Source: CAD feature listing. Evaluate the final solid. Frame: model axes, mm. A direction names the side the tool comes from. Give positions to 0.01 mm unless a question says otherwise; leave off trailing zeros. Loops run counter-clockwise (first coordinate to the right, second up) from the corner with the lowest first, then second, coordinate; pieces in that order, holes last.
from build123d import *

# Parameters (mm, degrees)
CROQUIS1_R              = 21
SALIENTE_EXTRUIR1_DEPTH = 40
SALIENTE_EXTRUIR2_DEPTH = 40
SALIENTE_EXTRUIR3_REACH = 77.493
CROQUIS3_R              = 13.5
CROQUIS3_R_2            = 10
CROQUIS7_R              = 8.227269221
CROQUIS7_R_2            = 6
CORTAR_EXTRUIR6_DEPTH   = 6
CROQUIS8_R              = 6
CORTAR_EXTRUIR7_DEPTH   = 72.223648425
CORTAR_EXTRUIR8_START   = -25
CORTAR_EXTRUIR8_DEPTH   = 25
CROQUIS12_R             = 9.55
CORTAR_EXTRUIR9_DEPTH   = 5.5


with BuildPart() as part:
    # Croquis1 → Saliente-Extruir1 (new body)
    with BuildSketch(Plane(origin=(0, 0, 0), x_dir=(1, 0, 0), z_dir=(0, 1, 0))):
        with Locations(Location((0, 0, 0), (0, 0, 270))):
            Circle(CROQUIS1_R)
    extrude(amount=SALIENTE_EXTRUIR1_DEPTH)

    # Croquis2 → Saliente-Extruir2 (add)
    with BuildSketch(Plane(origin=(0, 0, 0), x_dir=(1, 0, 0), z_dir=(0, 1, 0))):
        with BuildLine():
            Line((53.975127576, 8.110971331), (53.975127576, -11.889028669))
            Line((53.975127576, -11.889028669), (3.613793412, -20.686722727))
            ThreePointArc((3.613793412, -20.686722727), (20.98607707, -0.764571273), (5.109545014, 20.368911354))
            Line((5.109545014, 20.368911354), (53.975127576, 8.110971331))
        make_face()
    extrude(amount=SALIENTE_EXTRUIR2_DEPTH)

    # Croquis3 → Saliente-Extruir3 (add, up to next)
    with BuildSketch(Plane(origin=(5.109545014, 0, -20.368911354), x_dir=(-0.9699481597219111, 0, -0.24331166731597212), z_dir=(0.2433116673159721, 0, -0.969948159721911)), mode=Mode.PRIVATE) as saliente_extruir3_sk1:
        with Locations((0, 20)):
            Circle(CROQUIS3_R)
        with Locations((0, 20)):
            Circle(CROQUIS3_R_2, mode=Mode.SUBTRACT)
    saliente_extruir3_tool1 = extrude(saliente_extruir3_sk1.sketch, amount=-SALIENTE_EXTRUIR3_REACH, mode=Mode.PRIVATE) - part.part
    add(saliente_extruir3_tool1.solids().sort_by_distance((17.833482, 20, -17.177109))[0])

    # Croquis7 → Cortar-Extruir6 (cut)
    with BuildSketch(Plane.XZ):
        with Locations(Location((0, 0, 0), (0, 0, 270))):
            Circle(CROQUIS7_R)
        with Locations(Location((0, 0, 0), (0, 0, 270))):
            Circle(CROQUIS7_R_2, mode=Mode.SUBTRACT)
    extrude(amount=-CORTAR_EXTRUIR6_DEPTH, mode=Mode.SUBTRACT)

    # Croquis8 → Cortar-Extruir7 (cut, through all)
    with BuildSketch(Plane.XZ):
        with Locations(Location((0, 0, 0), (0, 0, 270))):
            Circle(CROQUIS8_R)
    extrude(amount=-CORTAR_EXTRUIR7_DEPTH, mode=Mode.SUBTRACT)

    # Croquis10 → Cortar-Extruir8 (cut)
    with BuildSketch(Plane(origin=(0, 40, 0), x_dir=(1, 0, 0), z_dir=(0, 1, 0)).offset(CORTAR_EXTRUIR8_START)):
        with BuildLine():
            Line((-5.995438853, 0.23390802), (-11.37823559, 0.424457107))
            Line((-11.37823559, 0.424457107), (-11.767631672, -10.575542893))
            Line((-11.767631672, -10.575542893), (30.232368328, -12.062327932))
            Line((30.232368328, -12.062327932), (30.62176441, -1.062327932))
            Line((30.62176441, -1.062327932), (5.996971268, -0.190619027))
            ThreePointArc((5.996971268, -0.190619027), (-0.212264906, -5.996244125), (-5.995438853, 0.23390802))
        make_face()
        with BuildLine():
            Line((-10.988839509, 11.424457107), (-11.37823559, 0.424457107))
            Line((-11.37823559, 0.424457107), (-5.995438853, 0.23390802))
            ThreePointArc((-5.995438853, 0.23390802), (0.116976243, 5.998859605), (6, 0))
            ThreePointArc((6, 0), (5.999242769, -0.095321543), (5.996971268, -0.190619027))
            Line((5.996971268, -0.190619027), (30.62176441, -1.062327932))
            Line((30.62176441, -1.062327932), (31.011160491, 9.937672068))
            Line((31.011160491, 9.937672068), (-10.988839509, 11.424457107))
        make_face()
    extrude(amount=CORTAR_EXTRUIR8_DEPTH, mode=Mode.SUBTRACT)

    # Croquis12 → Cortar-Extruir9 (cut)
    with BuildSketch(Plane(origin=(0, 15, 0), x_dir=(1, 0, 0), z_dir=(0, 1, 0))):
        with Locations(Location((0, 0, 0), (0, 0, 270))):
            Circle(CROQUIS12_R)
    extrude(amount=-CORTAR_EXTRUIR9_DEPTH, mode=Mode.SUBTRACT)


solid = part.part
1) Cut plane A-A (y = 35.5). Return loops of the section in (x, z).
Checks:
outline: (3.61, 20.69) arc R21 ccw (long way) to (5.11, -20.37) - (53.98, -8.11) - (53.98, 11.89) - close; hole (-11.77, 10.58) - (-10.99, -11.42) - (31.01, -9.94) - (30.23, 12.06) - close
2) Pull-direction query (Y, two-part tool) for faces 1 (the cylindrical face through (1.18, 19.86, -20.967)), 2 (the cylindrical face through (-4.823, 19.78, -21.863)), 3 (the flat face through (53.975, 20, 2)), 4 (the flat face through (-6.2, 9.5, -0.1)); classes: released by +Y, released by -Y, zero draft, split by the parting line, or undercut.
Checks:
face 1: undercut
face 2: undercut
face 3: zero draft
face 4: released by +Y
3) Reachability of faces 5 (the cylindrical face through (1.802, 7.726, -5.723)), 6 (the flat face through (-5, 6, -4)), 7 (the cylindrical face through (2.9, 12.3, 9.1)) from +Z, -Z, +X, -X, +Y, -Y: full face, straight path, thin tool, end or side. Return the list, or none.
Checks:
face 5: +Y, -Y
face 6: -Y
face 7: +Y
4) Cut plane C-C (y = 24). Return loops of the section in (x, z), and give its area (3 significant figures).
Checks:
outline: (-8.47, -19.21) - (-7.4, -23.51) - (-3.78, -22.6) - (-4.29, -20.56) arc R21 ccw to (5.11, -20.37) - (53.98, -8.11) - (53.98, 11.89) - (3.61, 20.69) arc R21 ccw to start; hole (-11.77, 10.58) - (-10.99, -11.42) - (31.01, -9.94) - (30.23, 12.06) - close
area: 1,480 mm2
5) Cut plane D-D (z = 13). Return loops of the section in (x, y), and give its area (3 significant figures).
Checks:
outline: (-16.49, 0) - (47.62, 0) - (47.62, 40) - (-16.49, 40) - close
area: 2,560 mm2
6) Ray query, probe 1 along X at (y, z) = (10.75, 0); probe 2 along X at (y, z) = (8.5, 0); probe 3 along Y at (x, z) = (5.5, -6.5). Return the intervals inside material, ascending.
Checks:
probe 1: x = -21 to -9.55, 9.55 to 53.98
probe 2: x = -21 to -6, 6 to 53.98
probe 3: y = 0 to 9.5
7) Contact query for flat-ended pins moving along their axis: P1, Ø8, axis at x = -2, z = -5, coming from the +Y side; P2, Ø2, axis at x = -2.5, z = -6, coming from the -Y side; P3, Ø1.5, axis at x = 17, z = -3.5, coming from the -Y side; P4, Ø1.5, axis at x = 37, y = 16.5, coming from the +Z side. Output: stop coordinate, or through.
Checks:
P1: stops at y = 9.5
P2: stops at y = 6
P3: stops at y = 0
P4: stops at z = 14.99
8) Cut plane B-B (z = 7). Return loops of the section in (x, y).
Checks:
outline: (-19.8, 0) - (-4.32, 0) - (-4.32, 6) - (4.32, 6) - (4.32, 0) - (53.98, 0) - (53.98, 40) - (30.41, 40) - (30.41, 15) - (6.5, 15) - (6.5, 9.5) - (-6.5, 9.5) - (-6.5, 15) - (-11.64, 15) - (-11.64, 40) - (-19.8, 40) - close
